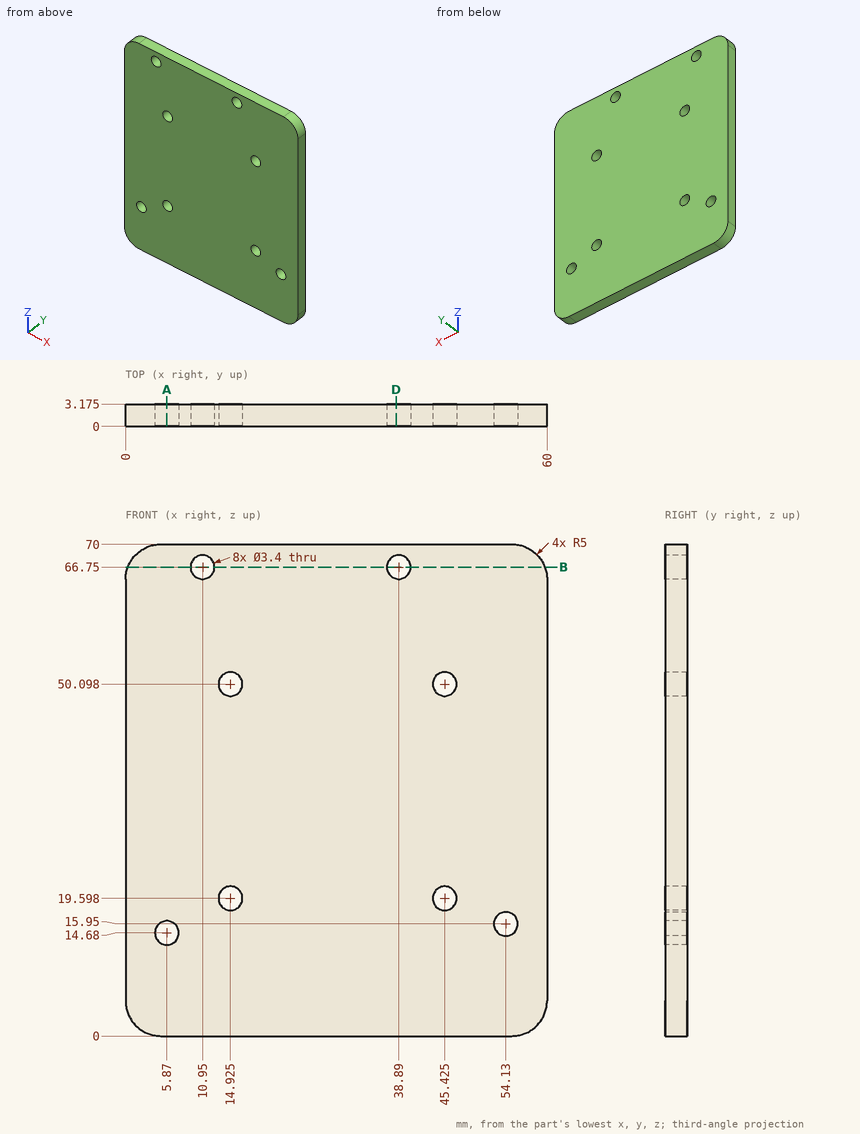
Print and shaded views of the part. All mm, measured from the part's lowest x, y and z. Give positions to 0.01 mm unless a question says otherwise; leave off trailing zeros. Loops run counter-clockwise (first coordinate to the right, second up) from the corner with the lowest first, then second, coordinate; pieces in that order, holes last. Notation, with made-up numbers: (-16, 48) - (38, 48) arc R32 cw to (38, 86) - close; hole circle Ø3 at (-3, -29). An arc over 180 degrees is marked (long way). One line per item, written item: value. Start each with the question number.
1. Probe L1, parallel to X at y = 2.25, z = 20; L2, parallel to Z at x = 5.87, y = 1.15; L3, parallel to X at y = 1.1, z = 14.68. List the from-to ranges inside material, lowest first. Write a range as from..to.
2. Slice it at D-D (x = 38.5). List the corners of the cut face in (y, z) (1 decimal).
3. Slice it at A-A (x = 5.87). List the corners of the cut face in (y, z) (1 decimal).
4. Slice it at B-B (z = 66.75). Give the number of separate pieces and of enclosed holes in the cut face, plus the area to 3 significant figures.
Solution:
1. L1: x = 0..13.27, 16.58..43.77, 47.08..60
1. L2: z = 0..12.98, 16.38..70
1. L3: x = 0..4.17, 7.57..53, 55.26..60
2. outline: (0, 0) - (3.2, 0) - (3.2, 65.1) - (0, 65.1) - close; (0, 68.4) - (3.2, 68.4) - (3.2, 70) - (0, 70) - close
3. outline: (0, 0) - (3.2, 0) - (3.2, 13) - (0, 13) - close; (0, 16.4) - (3.2, 16.4) - (3.2, 70) - (0, 70) - close
4. separate pieces: 3
4. enclosed holes: 0
4. area: 167 mm^2
